Read the model definition and answer for the solid it produces. Units are mm, in the model's axes. A direction names the side the tool comes from. Coordinates: 2 decimals unless noted, no trailing zeros. Write each loop counter-clockwise with the first axis right and the second up, starting at its lowest first coordinate (ties: lowest second). Pieces come first, ordered by that corner, then holes. Notation, with made-up numbers: (14.5, -26.75) -> (35.5, -26.75) arc R28 cw to (35.5, 2.25) -> close; hole circle Ø11 at (-33, 51). An arc over 180 degrees is marked (long way). Use CSV: the item, a comma, the result in double quotes.
from build123d import *

# Parameters (mm, degrees)
F1_DEPTH = 9
F3_DEPTH = 3
F4_R     = 2.25
F5_DEPTH = 25.4
F6_W     = 16.774124
F6_H     = 2.5
F6_W_2   = 6
F7_DEPTH = 25


with BuildPart() as f1:
    # F0 (on Top) → F1 (new body)
    with BuildSketch(Plane.XY):
        with BuildLine():
            ThreePointArc((13, 0), (6.5, 6.5), (0, 0))
            Line((0, 0), (0, -9))
            Line((0, -9), (13, -9))
            Line((13, -9), (13, 0))
        make_face()
    extrude(amount=F1_DEPTH)

    # F2 (on face) → F3 (cut)
    with BuildSketch(Plane.XY.offset(9)):
        Polygon((11.522947, -0.00093), (9.012279, 4.349535), (3.989331, 4.350465), (1.477053, 0.00093), (3.987721, -4.349535), (9.010669, -4.350465), align=None)
    extrude(amount=-F3_DEPTH, mode=Mode.SUBTRACT)

    # F4 (on face) → F5 (cut)
    with BuildSketch(Plane.XY.offset(9)):
        with Locations((6.5, 0)):
            Circle(F4_R)
    extrude(amount=-F5_DEPTH, mode=Mode.SUBTRACT)

    # F6 (on face) → F7 (cut)
    with BuildSketch(Plane(origin=(0, 0, 0), x_dir=(0, -1, 0), z_dir=(-1, 0, 0))):
        with Locations((-8.387062, 3.25)):
            Rectangle(F6_W, F6_H)
        with Locations((3, 3.25)):
            Rectangle(F6_W_2, F6_H)
    extrude(amount=-F7_DEPTH, mode=Mode.SUBTRACT)


solid = f1.part
1. For a pull along X with two mould halves and no side action, classify faces 4 (the flat face through (8, 2, 6)), 5 (the flat face through (6, -9, 4)), 6 (the flat face through (10.249, -2.206, 7.521)), 7 (the flat face through (13, -5, 5)) as pulls with the +X half, pulls with the -X half, needs draft (parallel to the pull), parting line crosses it, or undercut.
Solutions:
face 4,"undercut"
face 5,"needs draft"
face 6,"undercut"
face 7,"pulls with the +X half"
2. A cutting plane is placed at A-A (x = 6.5). Give the vertices of the cut face in (y, z).
Solutions:
outline,"(-9, 0) -> (-2.25, 0) -> (-2.25, 2) -> (-6, 2) -> (-6, 4.5) -> (-2.25, 4.5) -> (-2.25, 6) -> (-4.35, 6) -> (-4.35, 9) -> (-9, 9) -> close; (2.25, 0) -> (6.5, 0) -> (6.5, 2) -> (2.25, 2) -> close; (2.25, 4.5) -> (6.5, 4.5) -> (6.5, 9) -> (4.35, 9) -> (4.35, 6) -> (2.25, 6) -> close"
3. A tool of negligible diameter and unlimited length cuts with its end or side. For faces 1 (the flat face through (6, -3, 4.5)), 2 (the flat face through (6, -3, 0)), 3 (the flat face through (10.285, 2.144, 7.521)), from which of +Z, -Z, +X, -X, +Y, -Y can it reach the whole face along a straight path? Write none if from no direction.
Solutions:
face 1,"+X, -X, +Y"
face 2,"-Z, +X, -X, +Y, -Y"
face 3,"+Z"
4. A cutting plane is placed at C-C (z = 6.5). Give the vertices of the cut face in (x, y), and give its area (3 significant figures).
Solutions:
outline,"(0, -9) -> (13, -9) -> (13, 0) arc R6.5 ccw to (0, 0) -> close; hole (1.48, 0) -> (3.99, -4.35) -> (9.01, -4.35) -> (11.52, 0) -> (9.01, 4.35) -> (3.99, 4.35) -> close"
area,"118 mm^2"
5. Each of these flat-tipped pins is pushed along its axis until it touches: pin 1 Ø4.5 at (x, y) = (5.5, -1.5) entering from +Z; pin 2 Ø2 at (y, z) = (0.5, 4.5) entering from -X; pin 3 Ø0.9 at (x, z) = (5.5, 7) entering from +Y; pin 4 Ø1 at (x, z) = (9.5, 3) entering from +Y. Where does it stop, or does it pass through?
Solutions:
pin 1,"stops at z = 6"
pin 2,"stops at x = 0"
pin 3,"stops at y = 6.48"
pin 4,"stops at y = -6"
6. A cutting plane is placed at D-D (y = -3). Give the vertices of the cut face in (x, z), and give its area (3 significant figures).
Solutions:
outline,"(0, 0) -> (13, 0) -> (13, 2) -> (0, 2) -> close; (0, 4.5) -> (13, 4.5) -> (13, 9) -> (9.79, 9) -> (9.79, 6) -> (3.21, 6) -> (3.21, 9) -> (0, 9) -> close"
area,"64.8 mm^2"
7. Find the intervals of material crossed by line 1 along Z through (x, y) = (1, -3); line 2 along Y through (x, z) = (6.5, 0.7); line 3 along Z through (x, y) = (3, 1.75), in increasing order.
Solutions:
line 1,"z = 0 to 2, 4.5 to 9"
line 2,"y = -9 to -2.25, 2.25 to 6.5"
line 3,"z = 0 to 2, 4.5 to 6"
8. A cutting plane is placed at B-B (y = -0.5). Give the vertices of the cut face in (x, z), and give its area (3 significant figures).
Solutions:
outline,"(0, 0) -> (4.31, 0) -> (4.31, 2) -> (0, 2) -> close; (0, 4.5) -> (4.31, 4.5) -> (4.31, 6) -> (1.77, 6) -> (1.77, 9) -> (0, 9) -> close; (8.69, 0) -> (13, 0) -> (13, 2) -> (8.69, 2) -> close; (8.69, 4.5) -> (13, 4.5) -> (13, 9) -> (11.23, 9) -> (11.23, 6) -> (8.69, 6) -> close"
area,"40.7 mm^2"
